Autodesk Inventor part; units mm, degrees
ref_plane "YZ Plane" through (0, 0, 0) normal (1, 0, 0) x (0, 1, 0)
ref_plane "XZ Plane" through (0, 0, 0) normal (0, 1, 0) x (-1, 0, 0)
ref_plane "XY Plane" through (0, 0, 0) normal (0, 0, 1) x (1, 0, 0)
sketch "Sketch1" plane through (0, 0, 0) normal (0, 0, 1) x (1, 0, 0)
  line L0 (18, 7) -> (-162, 7)
  line L1 (-162, 0) -> (-162, 7)
  line L2 (18, 0) -> (-162, 0)
  line L3 (18, 7) -> (18, 0)
  line L4 (18, -6) -> (-162, -6)
  line L5 (-162, -13) -> (-162, -6)
  line L6 (-162, -13) -> (18, -13)
  line L7 (18, -6) -> (18, -13)
  line L8 (18, 0) -> (18, -6)
  line L9 (18, 7) -> (11, 7)
  line L10 (11, 7) -> (11, 0)
  line L11 (11, 0) -> (18, 0)
  line L12 (18, 0) -> (18, 7)
  line L13 (18, -6) -> (11, -6)
  line L14 (11, -6) -> (11, -13)
  line L15 (11, -13) -> (18, -13)
  line L16 (18, -13) -> (18, -6)
  line L17 (5, -13) -> (-2, -13)
  line L18 (-2, -13) -> (-2, -6)
  line L19 (-2, -6) -> (5, -6)
  line L20 (5, -6) -> (5, -13)
  line L21 (5, 0) -> (-2, 0)
  line L22 (-2, 0) -> (-2, 7)
  line L23 (-2, 7) -> (5, 7)
  line L24 (5, 7) -> (5, 0)
  line L25 (12, 1) -> (4, 1)
  line L26 (4, 1) -> (4, -7)
  line L27 (4, -7) -> (12, -7)
  line L28 (12, -7) -> (12, 1)
  point P0 (0, 0)
  point P1 (12, 0)
  point P2 (11, 1)
  point P3 (5, 1)
  point P4 (-2, 0)
  point P5 (4, 0)
  point P6 (4, -6)
  point P7 (-2, -13)
  point P8 (5, -7)
  point P9 (11, -7)
  point P10 (12, -6)
  dimension "d0" = 7
  dimension "d1" = 7
  dimension "d2" = 7
  dimension "d3" = 7
  dimension "d4" = 7
  dimension "d5" = 7
  dimension "d6" = 7
  dimension "d7" = 7
  dimension "d8" = 6
  dimension "d9" = 8
  dimension "d10" = 8
  dimension "d11" = 1
  dimension "d12" = 1
extrude "Extrusion1" add sketch "Sketch1" along normal blind 120 contours L3 L2 L28 L25 L10 L0 | L24 L25 L26 L2 L22 L0 | L25 L28 L2 L10 | L10 L2 L24 L25 | L28 L4 L26 L2 | L7 L6 L14 L27 L28 L4 | L24 L2 L26 L25 | L28 L27 L14 L4 | L14 L27 L20 L4 | L20 L27 L26 L4 | L6 L18 L4 L26 L27 L20
properties part number "zbar"
CAD build for the part. Positions are in the model's coordinates, mm. A direction names the side the tool comes from. Coordinates: 2 decimals unless noted, no trailing zeros. Write each loop counter-clockwise with the first axis right and the second up, starting at its lowest first coordinate (ties: lowest second). Pieces come first, ordered by that corner, then holes.
(1) Cut at D-D, the plane y = -2.75. List the corners of the cut face in (x, z).
(2) Drill centre lines: probe 1 along Y at (x, z) = (12.5, 24); probe 2 along X at (y, z) = (6, 68.5); probe 3 along X at (y, z) = (-5.5, 63.5). Where is each one in solid material? Low to high.
(3) Cut at B-B, the plane x = 3. List the corners of the cut face in (y, z).
(4) Cut at A-A, the plane y = 2.5. List the corners of the cut face in (x, z).
(5) Cut at C-C, the plane z = 36. List the corners of the cut face in (x, y).
(6) 3-axis set-ups, long thin cutter, end or side, ignore diameter. For faces 1 (the face through (5, -10, 59)), 2 (the face through (8, 1, 59)), 3 (the face through (1, 0, 59)), 4 (the face through (15, 0, 59)), 5 (the face through (1, -13, 59)): which of +Z, -Z, +X, -X, +Y, -Y reach the whole face in a straight line?
(7) Two-plate mould, pull along Y, no slides. Class faces 6 (the face through (14, -13, 59)), 7 (the face through (1, -6, 59)), 8 (the face through (15, -6, 59)), 9 (the face through (18, -9, 59)): +Y half, -Y half, draft (parallel to the pull), parting line (faces both ways), or undercut.
(8) Flat gauge pins, fed straight in: pin 1 (1.8 mm diameter, centred on y = -2, z = 81, fed in from -X); pin 2 (1.8 mm diameter, centred on x = 8.5, z = 77.5, fed in from +Y); pin 3 (6 mm diameter, centred on x = 6.5, z = 100.5, fed in from +Y); pin 4 (1.8 mm diameter, centred on y = -3, z = 82, fed in from +X). Where does each tip first touch, or does it go through?
Geometry says:
1. outline: (4, 0) - (12, 0) - (12, 120) - (4, 120) - close
2. probe 1: y = -13 to -6, 0 to 7
2. probe 2: x = -2 to 5, 11 to 18
2. probe 3: x = 4 to 12
3. outline: (-13, 0) - (-6, 0) - (-6, 120) - (-13, 120) - close; (0, 0) - (7, 0) - (7, 120) - (0, 120) - close
4. outline: (-2, 0) - (5, 0) - (5, 120) - (-2, 120) - close; (11, 0) - (18, 0) - (18, 120) - (11, 120) - close
5. outline: (-2, -13) - (5, -13) - (5, -7) - (11, -7) - (11, -13) - (18, -13) - (18, -6) - (12, -6) - (12, 0) - (18, 0) - (18, 7) - (11, 7) - (11, 1) - (5, 1) - (5, 7) - (-2, 7) - (-2, 0) - (4, 0) - (4, -6) - (-2, -6) - close
6. face 1: +Z, -Z, -Y
6. face 2: +Z, -Z, +Y
6. face 3: +Z, -Z, -X
6. face 4: +Z, -Z, +X
6. face 5: +Z, -Z, +X, -X, -Y
7. face 6: -Y half
7. face 7: undercut
7. face 8: undercut
7. face 9: draft
8. pin 1: stops at x = 4
8. pin 2: stops at y = 1
8. pin 3: stops at y = 7
8. pin 4: stops at x = 12
